Verification items for the finished model (mm, model axes). A direction names the side the tool comes from. Coordinates: 2 decimals unless noted, no trailing zeros. Loops run counter-clockwise (first coordinate to the right, second up) from the corner with the lowest first, then second, coordinate; pieces in that order, holes last.
Q1. Sectioned sample at A-A (y = 0). Enter the section's corners in (x, z).
Q2. Mould release check, pull along Y, two halves, no side actions. Record for faces 1 (the face through (0, 0, 28)), 2 (the face through (-3, 0, 6)), 3 (the face through (1, 3, 12)): +Y half, -Y half, draft (parallel to the pull), parting line (faces both ways), or undercut.
Q3. Material ranges on probe 1 along Z at (x, y) = (-1.75, 2.75); probe 2 along Y at (x, z) = (0, 34.5); probe 3 along Z at (x, y) = (1, -2.25), recorded low to high.
Q4. Sectioned sample at C-C (z = 21). Enter the section's corners in (x, y), then the cut area to 3 significant figures.
Q5. Go/stop test with flat-tipped pins: P1, Ø3, axis at x = 2, z = 35, coming from the +Y side; P2, Ø2, axis at y = -2, z = -3, coming from the +X side; P3, Ø0.8, axis at x = 0, y = -2.5, coming from the -Z side. Record where each tip stops, or that it passes through.
Q6. Access from +Z, -Z, +X, -X, +Y, -Y to the whole of each face (thin tool, end or side, straight path). Record for faces 4 (the face through (-2.86, -0.9, 37.86)), 5 (the face through (-2, 0.75, -3)), 6 (the face through (0, 3, -1.5)), 7 (the face through (2, -2, -3.5)), 8 (the face through (1, 3, 48)).
Q7. Sectioned sample at D-D (z = 37.5). Enter the section's corners in (x, y), then the cut area to 3 significant figures.
```python
from build123d import *

# Parameters (mm, degrees)
SKETCH1_R           = 3
BOSS_EXTRUDE1_DEPTH = 12
BOSS_EXTRUDE2_START = -3.5
SKETCH1_4_R         = 4
SKETCH1_4_R_2       = 3
BOSS_EXTRUDE2_DEPTH = 3.5
CUT_EXTRUDE1_DEPTH  = 2
FILLET1_R           = 0.5
CUT_EXTRUDE2_START  = -2
SKETCH2_3_R         = 1.25
CUT_EXTRUDE2_DEPTH  = 1
CUT_EXTRUDE2_DRAFT  = -20
FILLET2_R           = 0.5
BOSS_EXTRUDE3_START = 12
SKETCH1_5_R         = 4
BOSS_EXTRUDE3_DEPTH = 36
CUT_EXTRUDE3_START  = -20
SKETCH9_R           = 3
CUT_EXTRUDE3_DEPTH  = 20


with BuildPart() as part:
    # Sketch1 → Boss-Extrude1 (new body)
    with BuildSketch(Plane.XY):
        Circle(SKETCH1_R)
    extrude(amount=BOSS_EXTRUDE1_DEPTH)

    # Sketch1<4> → Boss-Extrude2 (add)
    # profile 1 of 2: a face of its own
    with BuildSketch(Plane.XY.offset(BOSS_EXTRUDE2_START)):
        Circle(SKETCH1_4_R)
        Circle(SKETCH1_4_R_2, mode=Mode.SUBTRACT)
    # profile 2 of 2: a face of its own
    with BuildSketch(Plane.XY.offset(BOSS_EXTRUDE2_START)):
        Circle(SKETCH1_4_R_2)
    extrude(amount=BOSS_EXTRUDE2_DEPTH)

    # Sketch2 → Cut-Extrude1 (cut)
    with BuildSketch(Plane(origin=(0, 0, -3.5), x_dir=(-1, 0, 0), z_dir=(0, 0, -1))):
        with BuildLine():
            ThreePointArc((0.75, 3.929058411), (0, 4), (-0.75, 3.929058411))
            Line((-0.75, 3.929058411), (-0.75, 1))
            ThreePointArc((-0.75, 1), (0, 1.25), (0.75, 1))
            Line((0.75, 1), (0.75, 3.929058411))
        make_face()
        with BuildLine():
            Line((-1, 0.75), (-3.929058411, 0.75))
            ThreePointArc((-3.929058411, 0.75), (-4, 0), (-3.929058411, -0.75))
            Line((-3.929058411, -0.75), (-1, -0.75))
            ThreePointArc((-1, -0.75), (-1.25, 0), (-1, 0.75))
        make_face()
        with BuildLine():
            ThreePointArc((4, 0), (3.98222511, 0.376673834), (3.929058411, 0.75))
            Line((3.929058411, 0.75), (1, 0.75))
            ThreePointArc((1, 0.75), (1.185854123, 0.395284708), (1.25, 0))
            ThreePointArc((1.25, 0), (1.185854123, -0.395284708), (1, -0.75))
            Line((1, -0.75), (3.929058411, -0.75))
            ThreePointArc((3.929058411, -0.75), (3.98222511, -0.376673834), (4, 0))
        make_face()
        with BuildLine():
            Line((-0.75, -1), (-0.75, -3.929058411))
            ThreePointArc((-0.75, -3.929058411), (0, -4), (0.75, -3.929058411))
            Line((0.75, -3.929058411), (0.75, -1))
            ThreePointArc((0.75, -1), (0, -1.25), (-0.75, -1))
        make_face()
        with BuildLine():
            ThreePointArc((0.75, 1), (0, 1.25), (-0.75, 1))
            Line((-0.75, 1), (-0.75, 0.75))
            Line((-0.75, 0.75), (-1, 0.75))
            ThreePointArc((-1, 0.75), (-1.25, 0), (-1, -0.75))
            Line((-1, -0.75), (-0.75, -0.75))
            Line((-0.75, -0.75), (-0.75, -1))
            ThreePointArc((-0.75, -1), (0, -1.25), (0.75, -1))
            Line((0.75, -1), (0.75, -0.75))
            Line((0.75, -0.75), (1, -0.75))
            ThreePointArc((1, -0.75), (1.185854123, -0.395284708), (1.25, 0))
            ThreePointArc((1.25, 0), (1.185854123, 0.395284708), (1, 0.75))
            Line((1, 0.75), (0.75, 0.75))
            Line((0.75, 0.75), (0.75, 1))
        make_face()
        with BuildLine():
            Line((-0.75, 0.75), (-0.75, 1))
            ThreePointArc((-0.75, 1), (-0.883883476, 0.883883476), (-1, 0.75))
            Line((-1, 0.75), (-0.75, 0.75))
        make_face()
        with BuildLine():
            ThreePointArc((1, 0.75), (0.883883476, 0.883883476), (0.75, 1))
            Line((0.75, 1), (0.75, 0.75))
            Line((0.75, 0.75), (1, 0.75))
        make_face()
        with BuildLine():
            ThreePointArc((0.75, -1), (0.883883476, -0.883883476), (1, -0.75))
            Line((1, -0.75), (0.75, -0.75))
            Line((0.75, -0.75), (0.75, -1))
        make_face()
        with BuildLine():
            Line((-0.75, -0.75), (-1, -0.75))
            ThreePointArc((-1, -0.75), (-0.883883476, -0.883883476), (-0.75, -1))
            Line((-0.75, -1), (-0.75, -0.75))
        make_face()
    extrude(amount=-CUT_EXTRUDE1_DEPTH, mode=Mode.SUBTRACT)

    # Fillet1
    fillet1_edges = [part.edges().sort_by_distance(p)[0] for p in [
        (-2.828427125, 2.828427125, -3.5),
        (-2.828427125, -2.828427125, -3.5),
        (2.828427125, -2.828427125, -3.5),
        (2.828427125, 2.828427125, -3.5),
    ]]
    fillet(fillet1_edges, radius=FILLET1_R)


with BuildPart() as cut_extrude2_tool:
    # Sketch2<3> → Cut-Extrude2 (with draft: the straight prism first)
    with BuildSketch(Plane(origin=(0, 0, -3.5), x_dir=(-1, 0, 0), z_dir=(0, 0, -1)).offset(CUT_EXTRUDE2_START)):
        Circle(SKETCH2_3_R)
    extrude(amount=-CUT_EXTRUDE2_DEPTH)
    # Cut-Extrude2: the draft: its side faces are tilted about the plane it starts from
    cut_extrude2_sides = [cut_extrude2_tool.faces().sort_by_distance(p)[0] for p in [
        (1.25, 0, -1),
    ]]
    draft(cut_extrude2_sides, Plane(origin=(0, 0, -3.5), x_dir=(-1, 0, 0), z_dir=(0, 0, -1)).offset(CUT_EXTRUDE2_START), CUT_EXTRUDE2_DRAFT)


with BuildPart() as part_1:
    add(part.part)

    # Cut-Extrude2: cut by cut_extrude2_tool
    add(cut_extrude2_tool.part, mode=Mode.SUBTRACT)

    # Fillet2
    fillet2_edges = [part_1.edges().sort_by_distance(p)[0] for p in [
        (0.886029766, 0, -0.5),
    ]]
    fillet(fillet2_edges, radius=FILLET2_R)

    # Sketch1<5> → Boss-Extrude3 (add)
    with BuildSketch(Plane.XY.offset(BOSS_EXTRUDE3_START)):
        Circle(SKETCH1_5_R)
    extrude(amount=BOSS_EXTRUDE3_DEPTH)

    # Sketch9 → Cut-Extrude3 (cut)
    with BuildSketch(Plane.XY.offset(48).offset(CUT_EXTRUDE3_START)):
        with Locations(Location((0, 0, 0), (0, 0, 180))):
            Circle(SKETCH9_R)
    extrude(amount=CUT_EXTRUDE3_DEPTH, mode=Mode.SUBTRACT)


solid = part_1.part
```
Geometry check:
1. outline: (-4, -1.5) - (-1.25, -1.5) - (-1.01, -0.83) arc R0.5 cw to (-0.54, -0.5) - (0.54, -0.5) arc R0.5 cw to (1.01, -0.83) - (1.25, -1.5) - (4, -1.5) - (4, 0) - (3, 0) - (3, 12) - (4, 12) - (4, 48) - (3, 48) - (3, 28) - (-3, 28) - (-3, 48) - (-4, 48) - (-4, 12) - (-3, 12) - (-3, 0) - (-4, 0) - close
2. face 1: undercut
2. face 2: parting line
2. face 3: draft
3. probe 1: z = -3.5 to 0, 12 to 48
3. probe 2: y = -4 to -3, 3 to 4
3. probe 3: z = -3.5 to 28
4. outline: circle Ø8 at (0, 0)
4. area: 50.3 mm2
5. P1: stops at y = 3.97
5. P2: stops at x = 3.87
5. P3: stops at z = -1.5
6. face 4: +Z
6. face 5: -Z, +X, -X
6. face 6: -Z, +Y, -Y
6. face 7: -Z, +X, -X, +Y, -Y
6. face 8: +Z, +X, -X, +Y, -Y
7. outline: circle Ø8 at (0, 0); hole circle Ø6 at (0, 0)
7. area: 22.0 mm2
